Check sheet for the modelled part. Datum: model origin and axes. Units: mm. A direction names the side the tool comes from. Round coordinates to 2 decimals unless told otherwise and drop trailing zeros. Write each loop counter-clockwise with the first axis right and the second up, starting at its lowest first coordinate (ties: lowest second). Pieces come first, ordered by that corner, then holes. Notation, with made-up numbers: M 40,-7.5 L 73,-7.5 A32 cw 73,28.5 Z; hole C 62.5,-34.5 d4. An arc over 180 degrees is marked long. Answer in a Markdown table with one row per item.
```python
from build123d import *

# Parameters (mm, degrees)
SKETCH_W        = 79.4
SKETCH_H        = 98.73
PAD_DEPTH       = 5
SKETCH002_W     = 69.4
SKETCH002_H     = 88.73
SKETCH002_W_2   = 65.4
SKETCH002_H_2   = 84.73
POCKET_DEPTH    = 2
SKETCH003_W     = 93.532375
SKETCH003_H     = 6
POCKET001_DEPTH = 2
SKETCH005_W     = 100.384567
SKETCH005_H     = 6
POCKET002_DEPTH = 2
SKETCH006_W     = 6
SKETCH006_H     = 113.061115
SKETCH006_H_2   = 111.176766
POCKET003_DEPTH = 2


with BuildPart() as part:
    # Sketch → Pad (new body)
    with BuildSketch(Plane.XY):
        Rectangle(SKETCH_W, SKETCH_H)
    extrude(amount=PAD_DEPTH)

    # Sketch002 → Pocket (cut)
    with BuildSketch(Plane(origin=(0, 0, 0), x_dir=(1, 0, 0), z_dir=(0, 0, -1))):
        Rectangle(SKETCH002_W, SKETCH002_H)
        Rectangle(SKETCH002_W_2, SKETCH002_H_2, mode=Mode.SUBTRACT)
    extrude(amount=-POCKET_DEPTH, mode=Mode.SUBTRACT)

    # Sketch003 (on Face16 of Pocket) → Pocket001 (cut)
    with BuildSketch(Plane(origin=(0, 0, 0), x_dir=(1, 0, 0), z_dir=(0, 0, -1))):
        with Locations((1.623375, 33.547611)):
            Rectangle(SKETCH003_W, SKETCH003_H)
    extrude(amount=-POCKET001_DEPTH, mode=Mode.SUBTRACT)

    # Sketch005 (on Face23 of Pocket001) → Pocket002 (cut)
    with BuildSketch(Plane(origin=(0, 0, 0), x_dir=(1, 0, 0), z_dir=(0, 0, -1))):
        with Locations((1.62792, -33.744774)):
            Rectangle(SKETCH005_W, SKETCH005_H)
    extrude(amount=-POCKET002_DEPTH, mode=Mode.SUBTRACT)

    # Sketch006 (on Face30 of Pocket002) → Pocket003 (cut)
    with BuildSketch(Plane(origin=(0, 0, 0), x_dir=(1, 0, 0), z_dir=(0, 0, -1))):
        with Locations((-25.195084, -4.192632)):
            Rectangle(SKETCH006_W, SKETCH006_H)
        with Locations((24.535048, -3.079151)):
            Rectangle(SKETCH006_W, SKETCH006_H_2)
    extrude(amount=-POCKET003_DEPTH, mode=Mode.SUBTRACT)


solid = part.part
```
1. Scan lines: L1, parallel to Y at x = 29.5, z = 1.6 (3 decimals); L2, parallel to X at y = 25.5, z = 0.5; L3, parallel to Z at x = -6, y = -42.5. Record each from-to range of solid material in increasing order.
Found:
| item | result |
|---|---|
| L1 | y = -49.365 to -44.365, -42.365 to -36.548, -30.548 to 30.745, 36.745 to 42.365, 44.365 to 49.365 |
| L2 | x = -39.7 to -34.7, -32.7 to -28.2, -22.2 to 21.54, 27.54 to 32.7, 34.7 to 39.7 |
| L3 | z = 2 to 5 |
2. Section check C-C, the plane x = -25. Record the cut outline in (y, z) (3 decimals).
Found:
| item | result |
|---|---|
| outline | M -49.365,2 L 49.365,2 L 49.365,5 L -49.365,5 Z |
3. Section check B-B, the plane x = 3.5. Record the cut outline in (y, z) (3 decimals), and give its area (3 significant figures).
Found:
| item | result |
|---|---|
| outline | M -49.365,0 L -44.365,0 L -44.365,2 L -42.365,2 L -42.365,0 L -36.548,0 L -36.548,2 L -30.548,2 L -30.548,0 L 30.745,0 L 30.745,2 L 36.745,2 L 36.745,0 L 42.365,0 L 42.365,2 L 44.365,2 L 44.365,0 L 49.365,0 L 49.365,5 L -49.365,5 Z |
| area | 462 mm2 |
4. Draft check along Y on faces 4 (the face through (-31, 44.365, 1)), 5 (the face through (35, 45, 0)), 6 (the face through (-31, -44.365, 1)). Enter one of: +Y half, -Y half, draft (parallel to the pull), parting line (faces both ways), or undercut.
Found:
| item | result |
|---|---|
| face 4 | undercut |
| face 5 | draft |
| face 6 | undercut |
5. Access from +Z, -Z, +X, -X, +Y, -Y to the whole of each face (thin tool, end or side, straight path). Record for faces 1 (the face through (-30, 36.745, 1)), 2 (the face through (-1, 42.365, 1)), 3 (the face through (21.535, 47, 1)).
Found:
| item | result |
|---|---|
| face 1 | -Z, +X, -X |
| face 2 | -Z |
| face 3 | -Z, +Y, -Y |
6. Section check A-A, the plane y = -27.5. Record the cut outline in (x, z), and give its area (3 significant figures).
Found:
| item | result |
|---|---|
| outline | M -39.7,0 L -34.7,0 L -34.7,2 L -32.7,2 L -32.7,0 L -28.2,0 L -28.2,2 L -22.2,2 L -22.2,0 L 21.54,0 L 21.54,2 L 27.54,2 L 27.54,0 L 32.7,0 L 32.7,2 L 34.7,2 L 34.7,0 L 39.7,0 L 39.7,5 L -39.7,5 Z |
| area | 365 mm2 |
